Source: CAD feature listing. Evaluate the final solid. Frame: model axes, mm. A direction names the side the tool comes from. Round coordinates to 2 decimals unless told otherwise and drop trailing zeros. Loops run counter-clockwise (first coordinate to the right, second up) from the corner with the lowest first, then second, coordinate; pieces in that order, holes last. Notation, with made-up numbers: M -2,80.25 L 55,80.25 A20 cw 55,86.25 Z; hole C -27,-26.5 d11. An arc over 180 degrees is marked long. One line per item, written item: value.
Autodesk Inventor part; units mm, degrees
ref_plane "YZ Plane" through (0, 0, 0) normal (1, 0, 0) x (0, 1, 0)
ref_plane "XZ Plane" through (0, 0, 0) normal (0, 1, 0) x (-1, 0, 0)
ref_plane "XY Plane" through (0, 0, 0) normal (0, 0, 1) x (1, 0, 0)
sketch "スケッチ1" plane through (0, 0, 0) normal (0, 0, 1) x (1, 0, 0)
  circle A0 centre (0, 0) radius 2.5
  dimension "d0" = 5
extrude "押し出し1" add sketch "スケッチ1" along normal blind 10
sketch "スケッチ2" plane through (0, 0, 0) normal (0, 0, -1) x (-1, 0, 0)
  line L0 (4.6188, 0) -> (2.3094, -4)
  line L1 (2.3094, -4) -> (-2.3094, -4)
  line L2 (-2.3094, -4) -> (-4.6188, 0)
  line L3 (-4.6188, 0) -> (-2.3094, 4)
  line L4 (-2.3094, 4) -> (2.3094, 4)
  line L5 (2.3094, 4) -> (4.6188, 0)
  point P0 (0, 0)
  point P1 (0, 0)
  dimension "d3" = 8
extrude "押し出し2" add sketch "スケッチ2" along normal blind 2.5
thread "ねじ1"
properties part number "ネジ六角ボルトm5,10" material "鋼、高強度、低合金"
1. Section query B-B (z = 4.75). Return the cut outline in (x, y), and give its area (3 significant figures).
Report:
outline: C 0,0 d5
area: 19.6 mm2
2. Reachability of faces 1 (the face through (3.448, -2.028, -1.232)), 2 (the face through (-2, 2, 0)) from +Z, -Z, +X, -X, +Y, -Y: full face, straight path, thin tool, end or side. Return the list, or none.
Report:
face 1: +Z, -Z, +X, -Y
face 2: +Z
3. Section query D-D (y = -3). Return the cut outline in (x, z), and give its area (3 significant figures).
Report:
outline: M -2.89,-2.5 L 2.89,-2.5 L 2.89,0 L -2.89,0 Z
area: 14.4 mm2
4. Section query A-A (x = 0). Return the cut outline in (y, z), and give its area (3 significant figures).
Report:
outline: M -4,-2.5 L 4,-2.5 L 4,0 L 2.5,0 L 2.5,10 L -2.5,10 L -2.5,0 L -4,0 Z
area: 70.0 mm2
5. Pin query (flat end, axial travel): pin 1 (4 mm diameter, centred on y = 2, z = 4.5, fed in from +X); pin 2 (1.5 mm diameter, centred on y = -2.5, z = 6.5, fed in from -X); pin 3 (1 mm diameter, centred on y = -1.5, z = 4.5, fed in from -X). Return the tip coordinate at first contact, or that it passes through.
Report:
pin 1: stops at x = 2.5
pin 2: stops at x = -1.79
pin 3: stops at x = -2.29
6. Ray query, line 1 (Z direction, x = -2.25, y = -3.5); line 2 (Y direction, x = -0.5, z = 7.25); line 3 (X direction, y = -1.25, z = 5). Return the intervals inside material, ascending. Write a range as [from, to].
Report:
line 1: z = [-2.5, 0]
line 2: y = [-2.45, 2.45]
line 3: x = [-2.17, 2.17]
7. Section query C-C (x = 1.5). Return the cut outline in (y, z), and give its area (3 significant figures).
Report:
outline: M -4,-2.5 L 4,-2.5 L 4,0 L 2,0 L 2,10 L -2,10 L -2,0 L -4,0 Z
area: 60.0 mm2
